Design review of the part built by this model. Coordinates are the model's own, in mm. A direction names the side the tool comes from. Give positions to 0.01 mm unless a question says otherwise; leave off trailing zeros. Loops run counter-clockwise (first coordinate to the right, second up) from the corner with the lowest first, then second, coordinate; pieces in that order, holes last. Notation, with made-up numbers: (-31, 61.5) - (-8, 61.5) arc R29 cw to (-8, 89.5) - close; hole circle Ø6 at (58, 6). An arc over 180 degrees is marked (long way). One line per item, written item: value. Start each with the question number.
```python
from build123d import *

# Parameters (mm, degrees)
EXTRUDE_1_DEPTH     = 5
SKETCH_3_R          = 2.75
CUT_EXTRUDE_1_DEPTH = 5
SKETCH_4_W          = 25
SKETCH_4_H          = 5
EXTRUDE_2_DEPTH     = 5
SKETCH_5_R          = 1.55
CUT_EXTRUDE_2_DEPTH = 5
FILLET_1_R          = 30
FILLET_2_R          = 1


with BuildPart() as part:
    # 草图1 → 凸台-拉伸1 (new body)
    with BuildSketch(Plane(origin=(0, 0, 0), x_dir=(1, 0, 0), z_dir=(0, 1, 0))):
        Polygon((-20, 100), (20, 100), (20, 11.547005384), (87.5, -27.424137787), (107.5, -38.97114317), (107.5, -90), (67.5, -90), (67.5, -62.065153938), (0, -23.094010768), (-67.5, -62.065153938), (-67.5, -90), (-107.5, -90), (-107.5, -38.97114317), (-87.5, -27.424137787), (-20, 11.547005384), align=None)
    extrude(amount=EXTRUDE_1_DEPTH)

    # 草图3 → 切除-拉伸1 (cut)
    with BuildSketch(Plane(origin=(0, 5, 0), x_dir=(1, 0, 0), z_dir=(0, 1, 0))):
        with Locations(Location((0, 37.498899984, 0), (0, 0, 270))):
            Circle(SKETCH_3_R)
        with Locations(Location((32.475, -18.749449992, 0), (0, 0, 270))):
            Circle(SKETCH_3_R)
        with Locations(Location((-32.475, -18.749449992, 0), (0, 0, 270))):
            Circle(SKETCH_3_R)
    extrude(amount=-CUT_EXTRUDE_1_DEPTH, mode=Mode.SUBTRACT)

    # 草图4 → 凸台-拉伸2 (add)
    with BuildSketch(Plane(origin=(0, 5, 0), x_dir=(1, 0, 0), z_dir=(0, 1, 0))):
        with Locations((-87.5, -92.5)):
            Rectangle(SKETCH_4_W, SKETCH_4_H)
        with Locations((87.5, -92.5)):
            Rectangle(SKETCH_4_W, SKETCH_4_H)
        with Locations((0, 102.5)):
            Rectangle(SKETCH_4_W, SKETCH_4_H)
    extrude(amount=-EXTRUDE_2_DEPTH)

    # 草图5 → 切除-拉伸2 (cut)
    with BuildSketch(Plane(origin=(0, 5, 0), x_dir=(1, 0, 0), z_dir=(0, 1, 0))):
        with Locations((14.05, 100)):
            Circle(SKETCH_5_R)
        with Locations((-14.05, 100)):
            Circle(SKETCH_5_R)
        with Locations((-73.45, -90)):
            Circle(SKETCH_5_R)
        with Locations((-101.55, -90)):
            Circle(SKETCH_5_R)
        with Locations((101.55, -90)):
            Circle(SKETCH_5_R)
        with Locations((73.45, -90)):
            Circle(SKETCH_5_R)
    extrude(amount=-CUT_EXTRUDE_2_DEPTH, mode=Mode.SUBTRACT)

    # 圆角1
    fillet_1_edges = [part.edges().sort_by_distance(p)[0] for p in [
        (-20, 2.5, -11.547005384),
        (20, 2.5, -11.547005384),
        (107.5, 2.5, 38.97114317),
        (67.5, 2.5, 62.065153938),
        (0, 2.5, 23.094010768),
        (-67.5, 2.5, 62.065153938),
        (-107.5, 2.5, 38.97114317),
    ]]
    fillet(fillet_1_edges, radius=FILLET_1_R)

    # 圆角2
    fillet_2_edges = [part.edges().sort_by_distance(p)[0] for p in [
        (-20, 2.5, -100),
        (20, 2.5, -100),
        (107.5, 2.5, 90),
        (67.5, 2.5, 90),
        (-67.5, 2.5, 90),
        (-107.5, 2.5, 90),
    ]]
    fillet(fillet_2_edges, radius=FILLET_2_R)


solid = part.part
```
(1) Take a section at A-A on z = -75.5. State the section outline as (x, y) points.
(2) For pin 1 Ø1.7 at (x, y) = (104.5, 2) entering from +Z; pin 2 Ø1 at (x, y) = (-51.5, 1.5) entering from +Z; pin 3 Ø3 at (x, y) = (66.5, 3) entering from +Z; pin 4 Ø5 at (x, z) = (64.5, 52) entering from -Y, all flat-tipped, find the tip position at first contact; note any pin that passes through.
(3) To check wall thickness, follow L1, parallel to X at y = 1.15, z = 86; L2, parallel to X at y = 4.4, z = -55; L3, parallel to X at y = 3, z = 39. State the ranges of each line that lie inside material, in increasing order. Write a range as from..to.
(4) Take a section at B-B on x = -84. State the section outline as (y, z) points.
(5) Machinability: for faces 1 (the flat face through (20, 2, -64)), 2 (the flat face through (1, 0, 17)), 3 (the flat face through (67.5, 2, 84)), 4 (the flat face through (87, 3, 95)), 5 (the flat face through (-12.5, 3, -102)), which of the approach directions +Z, -Z, +X, -X, +Y, -Y give a long, thin tool a straight path to every point of the face, cutting with its end or side? Answer none if there is none.
(6) Draft analysis for pull direction X (two halves, no side actions). For faces 6 (the cylindrical face through (-0.22, 2.535, 27.736)), 7 (the flat face through (-100, 3, 93)), 8 (the cylindrical face through (24.13, 2.54, -13.68)), state which applies: pulls with the +X half, pulls with the -X half, needs draft (parallel to the pull), parting line crosses it, or undercut.
Here are the results:
1. outline: (-20, 0) - (20, 0) - (20, 5) - (-20, 5) - close
2. pin 1: z = 90
2. pin 2: z = 53.12
2. pin 3: z = 89.87
2. pin 4: y = 0
3. L1: -107.5..-67.5, 67.5..107.5
3. L2: -20..20
3. L3: -102.02..-27.55, 27.55..102.02
4. outline: (0, 25.4) - (5, 25.4) - (5, 95) - (0, 95) - close
5. face 1: -Z, +X, +Y, -Y
5. face 2: +Z, -Z, +X, -X, -Y
5. face 3: +Z, +Y, -Y
5. face 4: +Z, +X, -X, +Y, -Y
5. face 5: -Z, -X, +Y, -Y
6. face 6: undercut
6. face 7: pulls with the -X half
6. face 8: pulls with the +X half
